Autodesk Inventor part; units mm, degrees
ref_plane "YZ Plane" through (0, 0, 0) normal (1, 0, 0) x (0, 1, 0)
ref_plane "XZ Plane" through (0, 0, 0) normal (0, 1, 0) x (-1, 0, 0)
ref_plane "XY Plane" through (0, 0, 0) normal (0, 0, 1) x (1, 0, 0)
sketch "Sketch1" plane through (0, 0, 0) normal (0, 1, 0) x (-1, 0, 0)
  line L0 (0, 0) -> (-320, 0)
  line L1 (-320, 0) -> (-320, -160)
  line L2 (-320, -160) -> (0, -160)
  line L3 (0, -160) -> (0, 0)
  line L4 (-2.5, -157.5) -> (-317.5, -157.5)
  line L5 (-317.5, -157.5) -> (-317.5, -2.5)
  line L6 (-317.5, -2.5) -> (-2.5, -2.5)
  line L7 (-2.5, -2.5) -> (-2.5, -157.5)
  line L8 (-32.5, -142.5) -> (-52.5, -142.5)
  line L9 (-52.5, -142.5) -> (-52.5, -132.5)
  line L10 (-52.5, -132.5) -> (-32.5, -132.5)
  line L11 (-32.5, -132.5) -> (-32.5, -142.5)
  line L12 (-287.5, -142.5) -> (-267.5, -142.5)
  line L13 (-267.5, -142.5) -> (-267.5, -132.5)
  line L14 (-267.5, -132.5) -> (-287.5, -132.5)
  line L15 (-287.5, -132.5) -> (-287.5, -142.5)
  line L16 (-166.25, -142.5) -> (-153.75, -142.5)
  line L17 (-153.75, -142.5) -> (-153.75, -132.5)
  line L18 (-153.75, -132.5) -> (-166.25, -132.5)
  line L19 (-166.25, -132.5) -> (-166.25, -142.5)
  line L20 (-2.5, -80) -> (-317.5, -80)
  line L21 (-32.5, -17.5) -> (-52.5, -17.5)
  line L22 (-52.5, -17.5) -> (-52.5, -27.5)
  line L23 (-52.5, -27.5) -> (-32.5, -27.5)
  line L24 (-32.5, -27.5) -> (-32.5, -17.5)
  line L25 (-287.5, -17.5) -> (-267.5, -17.5)
  line L26 (-267.5, -17.5) -> (-267.5, -27.5)
  line L27 (-267.5, -27.5) -> (-287.5, -27.5)
  line L28 (-287.5, -27.5) -> (-287.5, -17.5)
  line L29 (-166.25, -17.5) -> (-153.75, -17.5)
  line L30 (-153.75, -17.5) -> (-153.75, -27.5)
  line L31 (-153.75, -27.5) -> (-166.25, -27.5)
  line L32 (-166.25, -27.5) -> (-166.25, -17.5)
  point P0 (-32.5, -137.5)
  point P1 (-42.5, -142.5)
  point P2 (-277.5, -142.5)
  point P3 (-287.5, -137.5)
  point P4 (-52.5, -137.5)
  point P5 (-267.5, -137.5)
  point P6 (-160, -142.5)
  point P7 (-32.5, -22.5)
  point P8 (-42.5, -17.5)
  point P9 (-277.5, -17.5)
  point P10 (-287.5, -22.5)
  point P11 (-52.5, -22.5)
  point P12 (-267.5, -22.5)
  point P13 (-160, -17.5)
  dimension "d0" = 320
  dimension "d1" = 160
  dimension "d2" = 2.5
  dimension "d7" = 30
  dimension "d8" = 15
  dimension "d9" = 20
  dimension "d10" = 10
  dimension "d11" = 20
  dimension "d12" = 10
  dimension "d13" = 15
  dimension "d14" = 30
  dimension "d16" = 215
  dimension "d18" = 10
  dimension "d19" = 12.5
  dimension "d23" = 160
  dimension "d25" = 15
extrude "Extrusion1" add sketch "Sketch1" along normal blind 2 contours L3 L2 L1 L0 | L4 L5 L20 L7 | L20 L5 L6 L7
sketch "Sketch2" plane through (0, 2, 0) normal (0, 1, 0) x (1, 0, 0)
  line L0 (320, 0) -> (320, 160)
  line L1 (320, 160) -> (0, 160)
  line L2 (0, 160) -> (0, 0)
  line L3 (0, 0) -> (320, 0)
  line L4 (32.5, 142.5) -> (52.5, 142.5)
  line L5 (52.5, 142.5) -> (52.5, 132.5)
  line L6 (52.5, 132.5) -> (32.5, 132.5)
  line L7 (32.5, 132.5) -> (32.5, 142.5)
  line L8 (287.5, 142.5) -> (287.5, 132.5)
  line L9 (287.5, 132.5) -> (267.5, 132.5)
  line L10 (267.5, 132.5) -> (267.5, 142.5)
  line L11 (267.5, 142.5) -> (287.5, 142.5)
  line L12 (166.25, 142.5) -> (166.25, 132.5)
  line L13 (166.25, 132.5) -> (153.75, 132.5)
  line L14 (153.75, 132.5) -> (153.75, 142.5)
  line L15 (153.75, 142.5) -> (166.25, 142.5)
  line L16 (52.5, 17.5) -> (32.5, 17.5)
  line L17 (32.5, 17.5) -> (32.5, 27.5)
  line L18 (32.5, 27.5) -> (52.5, 27.5)
  line L19 (52.5, 27.5) -> (52.5, 17.5)
  line L20 (267.5, 17.5) -> (267.5, 27.5)
  line L21 (267.5, 27.5) -> (287.5, 27.5)
  line L22 (287.5, 27.5) -> (287.5, 17.5)
  line L23 (287.5, 17.5) -> (267.5, 17.5)
  line L24 (166.25, 27.5) -> (166.25, 17.5)
  line L25 (166.25, 17.5) -> (153.75, 17.5)
  line L26 (153.75, 17.5) -> (153.75, 27.5)
  line L27 (153.75, 27.5) -> (166.25, 27.5)
  line L28 (2.5, 2.5) -> (2.5, 157.5)
  line L29 (2.5, 157.5) -> (317.5, 157.5)
  line L30 (317.5, 157.5) -> (317.5, 2.5)
  line L31 (317.5, 2.5) -> (2.5, 2.5)
  dimension "d26" = 2.5
extrude "Extrusion2" add sketch "Sketch2" along normal blind 10 and the other way blind 30 contours L3 L2 L1 L0
sketch "Sketch3" plane through (0, -28, 0) normal (0, -1, 0) x (1, 0, 0)
  line L0 (0, 0) -> (0, -160)
  line L1 (0, -160) -> (320, -160)
  line L2 (320, -160) -> (320, 0)
  line L3 (320, 0) -> (0, 0)
properties part number "led_spectrum_frame"
The model under review builds one solid part; all positions refer to its coordinate system, in mm. A direction names the side the tool comes from. Give positions to 0.01 mm unless a question says otherwise; leave off trailing zeros. Write each loop counter-clockwise with the first axis right and the second up, starting at its lowest first coordinate (ties: lowest second). Pieces come first, ordered by that corner, then holes. Notation, with made-up numbers: (19, 42.5) - (68, 42.5) arc R12 cw to (68, 52.5) - close; hole circle Ø8 at (-3, 38). An arc over 180 degrees is marked (long way). Answer in a Markdown table with one row per item. Add a question column.
1. Insertion check: P1, Ø8, axis at x = 228, z = -68, coming from the +Y side; P2, Ø3, axis at x = 38, z = -135.5, coming from the +Y side. Each pin has a flat end and moves straight along its axis. Give the tip position at first contact, or say it passes through.
2. Wall thickness on line 1 along X through (y, z) = (-23, -10.5); line 2 along Z through (x, y) = (209, -10.5); line 3 along Y through (x, z) = (82, -123): over which ranges is each line inside the solid? List them lowest first. Write a range as [from, to].
3. We need section C-C on z = -70. Write out the cut boundary in (x, y), then the cut area to 3 significant figures.
4. Draft analysis for pull direction Z (two halves, no side actions). For faces 1 (the flat face through (158, -8, 0)), 2 (the flat face through (320, -8, -79)), 3 (the flat face through (162, 2, -79)), state which applies: +Z half, -Z half, draft (parallel to the pull), parting line (faces both ways), or undercut.
5. We need section A-A on x = 198. Write out the cut boundary in (y, z).
6. We need section B-B on y = -7. Write out the cut boundary in (x, z).
7. Tool access review of faces 4 (the flat face through (0, -8, -81)), 5 (the flat face through (162, -14, -2.5)), 6 (the flat face through (158, 7, -157.5)): name each direction out of +Z, -Z, +X, -X, +Y, -Y from which nothing blocks a thin tool from reaching the whole face with its end or side.
Ans:
| question | item | result |
|---|---|---|
| 1 | P1 | stops at y = 2 |
| 1 | P2 | passes through |
| 2 | line 1 | x = [0, 2.5], [317.5, 320] |
| 2 | line 2 | z = [-160, -157.5], [-2.5, 0] |
| 2 | line 3 | y = [0, 2] |
| 3 | outline | (0, -28) - (2.5, -28) - (2.5, 0) - (317.5, 0) - (317.5, -28) - (320, -28) - (320, 12) - (317.5, 12) - (317.5, 2) - (2.5, 2) - (2.5, 12) - (0, 12) - close |
| 3 | area | 830 mm^2 |
| 4 | face 1 | +Z half |
| 4 | face 2 | draft |
| 4 | face 3 | undercut |
| 5 | outline | (-28, -160) - (12, -160) - (12, -157.5) - (2, -157.5) - (2, -2.5) - (12, -2.5) - (12, 0) - (-28, 0) - (-28, -2.5) - (0, -2.5) - (0, -157.5) - (-28, -157.5) - close |
| 6 | outline | (0, -160) - (320, -160) - (320, 0) - (0, 0) - close; hole (2.5, -157.5) - (317.5, -157.5) - (317.5, -2.5) - (2.5, -2.5) - close |
| 7 | face 4 | +Z, -Z, -X, +Y, -Y |
| 7 | face 5 | -Y |
| 7 | face 6 | +Y |
